from build123d import *

# Parameters (mm, degrees)
SKETCH1_R           = 5
BOSS_EXTRUDE1_DEPTH = 0.2
SKETCH2_W           = 15
SKETCH2_H           = 15
BOSS_EXTRUDE2_DEPTH = 0.4
FILLET1_R           = 2.5


with BuildPart() as part:
    # Sketch1 → Boss-Extrude1 (new body)
    with BuildSketch(Plane(origin=(0, 0, 0), x_dir=(1, 0, 0), z_dir=(0, 1, 0))):
        Circle(SKETCH1_R)
    extrude(amount=BOSS_EXTRUDE1_DEPTH)

    # Sketch2 → Boss-Extrude2 (add)
    with BuildSketch(Plane(origin=(0, 0.2, 0), x_dir=(1, 0, 0), z_dir=(0, 1, 0))):
        Rectangle(SKETCH2_W, SKETCH2_H)
    extrude(amount=BOSS_EXTRUDE2_DEPTH)

    # Fillet1
    fillet1_edges = [part.edges().sort_by_distance(p)[0] for p in [
        (7.5, 0.4, 7.5),
        (7.5, 0.4, -7.5),
        (-7.5, 0.4, -7.5),
        (-7.5, 0.4, 7.5),
    ]]
    fillet(fillet1_edges, radius=FILLET1_R)


solid = part.part
Could you check a few things on this model? Use its own coordinates, in mm. A direction names the side the tool comes from. Coordinates: 2 decimals unless noted, no trailing zeros. Order: outer loops, then holes, each group sorted by start corner. A loop starts at its lowest first (then second) coordinate and runs counter-clockwise, first axis right, second up. Notation, with made-up numbers: (-2.5, 86.5) -> (3.5, 86.5) arc R13 ccw to (3.5, 100.5) -> close; hole circle Ø6 at (-21, -0.75). An arc over 180 degrees is marked (long way). One line per question, with ' | ' between items.
Q1. Imagine slicing it at C-C on x = 6. Please give me the cut outline in (y, z).
Return value:
outline: (0.2, -7.29) -> (0.6, -7.29) -> (0.6, 7.29) -> (0.2, 7.29) -> close
Q2. Imagine slicing it at A-A on z = 0. Please give me the cut outline in (x, y).
Return value:
outline: (-7.5, 0.2) -> (-5, 0.2) -> (-5, 0) -> (5, 0) -> (5, 0.2) -> (7.5, 0.2) -> (7.5, 0.6) -> (-7.5, 0.6) -> close
Q3. If I drill on L1, parallel to Y at x = 5.25, z = -1; L2, parallel to Z at x = -6.25, y = 0.35; L3, parallel to Z at x = -6, y = 0.3, over which ranges is the centre line in solid material (lowest first)?
Return value:
L1: 0.2 to 0.6 | L2: -7.17 to 7.17 | L3: -7.29 to 7.29
Q4. On a 3-axis mill with a long thin cutter (end or side, diameter ignored), from which of +Z, -Z, +X, -X, +Y, -Y can I reach the whole of each face in a straight line? I mean faces 1 (the face through (2, 0.2, 5)), 2 (the face through (-6.787, 0.403, -6.748)). Say none if no direction works.
Return value:
face 1: -Y | face 2: -Z, -X, +Y, -Y
Q5. Imagine slicing it at D-D on x = -6.25. Please give me the cut outline in (y, z), and give its area (3 significant figures).
Return value:
outline: (0.2, -7.17) -> (0.6, -7.17) -> (0.6, 7.17) -> (0.2, 7.17) -> close | area: 5.73 mm²
Q6. Imagine slicing it at B-B on x = 0. Please give me the cut outline in (y, z), and give its area (3 significant figures).
Return value:
outline: (0, -5) -> (0.2, -5) -> (0.2, -7.5) -> (0.6, -7.5) -> (0.6, 7.5) -> (0.2, 7.5) -> (0.2, 5) -> (0, 5) -> close | area: 8.00 mm²
